```python
from build123d import *

# Parameters (mm, degrees)
SKETCH4_R           = 2.54
BOSS_EXTRUDE1_DEPTH = 3.175


with BuildPart() as part:
    # Sketch4 → Boss-Extrude1 (new body)
    with BuildSketch(Plane.XY):
        Polygon((0, 0), (12.7, 0), (12.7, 15.24), (9.525, 18.529765797), (3.175, 18.529765797), (0, 15.24), align=None)
        with Locations((6.35, 10.909765797)):
            Circle(SKETCH4_R, mode=Mode.SUBTRACT)
    boss_extrude1 = extrude(amount=BOSS_EXTRUDE1_DEPTH)

    # Mirror1: Boss-Extrude1 across plane
    add(boss_extrude1.mirror(Plane.ZX))


solid = part.part
```
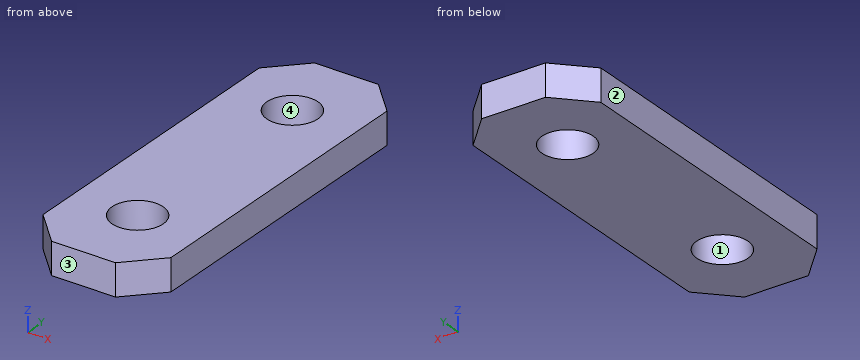
Source: CAD feature listing. Evaluate the final solid. Frame: model axes, mm. Face numbers are marked on the shaded views. Give positions to 0.01 mm unless a question says otherwise; leave off trailing zeros. Loops run counter-clockwise (first coordinate to the right, second up) from the corner with the lowest first, then second, coordinate; pieces in that order, holes last. Notation, with made-up numbers: (41.25, 84) -> (84.25, 84) arc R9 cw to (84.25, 96) -> close; hole circle Ø8 at (41, -38). An arc over 180 degrees is marked (long way). Put each result on its own line as item: value. Start each with the question number.
1) Contact query for a flat-ended pin moving along its axis: P1, Ø1.5, axis at x = 2, z = 2, coming from the -Y side. Output: stop coordinate, or through.
2) Cut plane D-D (x = 4.5). Return loops of the section in (y, z) (3 decimals).
3) Cut plane B-B (x = 6.35). Return loops of the section in (y, z) (3 decimals), then the cut area to 3 significant figures.
4) Cut plane C-C (z = 2.4). Return loops of the section in (x, y) (3 decimals), then the cut area to 3 significant figures.
5) Draft query along Y for the marked faces 1, 2, 3 and 4. Return one class per face: released by +Y, released by -Y, zero draft, split by the parting line, or undercut.
6) Cut plane A-A (y = -13). Return loops of the section in (x, z) (3 decimals), then the cut area to 3 significant figures.
7) Material intervals for probe 1 along Y at (x, z) = (6.35, 0.95); probe 2 along Y at (x, z) = (5.25, 2); probe 3 along X at (y, z) = (11, 2.4), sorted ascending.
Results are:
1. P1: stops at y = -18.09
2. outline: (-18.53, 0) -> (-12.65, 0) -> (-12.65, 3.175) -> (-18.53, 3.175) -> close; (-9.169, 0) -> (9.169, 0) -> (9.169, 3.175) -> (-9.169, 3.175) -> close; (12.65, 0) -> (18.53, 0) -> (18.53, 3.175) -> (12.65, 3.175) -> close
3. outline: (-18.53, 0) -> (-13.45, 0) -> (-13.45, 3.175) -> (-18.53, 3.175) -> close; (-8.37, 0) -> (8.37, 0) -> (8.37, 3.175) -> (-8.37, 3.175) -> close; (13.45, 0) -> (18.53, 0) -> (18.53, 3.175) -> (13.45, 3.175) -> close
3. area: 85.4 mm2
4. outline: (0, -15.24) -> (3.175, -18.53) -> (9.525, -18.53) -> (12.7, -15.24) -> (12.7, 15.24) -> (9.525, 18.53) -> (3.175, 18.53) -> (0, 15.24) -> close; hole circle Ø5.08 at (6.35, -10.91); hole circle Ø5.08 at (6.35, 10.91)
4. area: 409 mm2
5. face 1: undercut
5. face 2: zero draft
5. face 3: released by -Y
5. face 4: undercut
6. outline: (0, 0) -> (4.907, 0) -> (4.907, 3.175) -> (0, 3.175) -> close; (7.793, 0) -> (12.7, 0) -> (12.7, 3.175) -> (7.793, 3.175) -> close
6. area: 31.2 mm2
7. probe 1: y = -18.53 to -13.45, -8.37 to 8.37, 13.45 to 18.53
7. probe 2: y = -18.53 to -13.2, -8.62 to 8.62, 13.2 to 18.53
7. probe 3: x = 0 to 3.81, 8.89 to 12.7
